from build123d import *

# Parameters (mm, degrees)
SKETCH_R   = 3
SKETCH_R_2 = 1.5
PAD_DEPTH  = 1.5


with BuildPart() as part:
    # Sketch → Pad (new body)
    with BuildSketch(Plane.XY):
        with BuildLine():
            Line((70, 0), (0, 0))
            Line((0, 0), (0, 50))
            Line((0, 50), (70, 50))
            Line((70, 50), (70, 40))
            ThreePointArc((70, 40), (55, 25), (70, 10))
            Line((70, 0), (70, 10))
        make_face()
        with Locations((28, 25)):
            Circle(SKETCH_R, mode=Mode.SUBTRACT)
        with Locations((49, 25)):
            Circle(SKETCH_R_2, mode=Mode.SUBTRACT)
        with Locations((59.5, 43.19)):
            Circle(SKETCH_R_2, mode=Mode.SUBTRACT)
        with Locations((59.5, 6.81)):
            Circle(SKETCH_R_2, mode=Mode.SUBTRACT)
    extrude(amount=PAD_DEPTH)


solid = part.part
CAD build for the part. Positions are in the model's coordinates, mm. Coordinates: 2 decimals unless noted, no trailing zeros. Write each loop counter-clockwise with the first axis right and the second up, starting at its lowest first coordinate (ties: lowest second). Pieces come first, ordered by that corner, then holes. Notation, with made-up numbers: M -18.5,83 L 19.5,83 A25 ccw 19.5,103 Z; hole C 11,28.5 d4. An arc over 180 degrees is marked long. Return JSON: item names as keys, results as strings.
Item 1: Slice it at B-B, the plane y = 6.81. Write the cut outline in (x, z), and give its area (4 significant figures).
Findings below:
{"outline": "M 0,0 L 58,0 L 58,1.5 L 0,1.5 Z; M 61,0 L 70,0 L 70,1.5 L 61,1.5 Z", "area": "100.5 mm2"}
Item 2: Probe line 1 (Y direction, x = 49, z = 0.65); line 2 (Y direction, x = 59.5, z = 0.85); line 3 (Y direction, x = 63.5, z = 0.55). List the from-to ranges inside material, lowest first. Write a range as from..to.
Findings below:
{"line 1": "y = 0..23.5, 26.5..50", "line 2": "y = 0..5.31, 8.31..14.29, 35.71..41.69, 44.69..50", "line 3": "y = 0..11.48, 38.52..50"}
Item 3: Two-plate mould, pull along Y, no slides. Class faces 1 (the flat face through (35, 50, 1)), 2 (the flat face through (35, 25, 0)), 3 (the cylindrical face through (60.93, 7.26, 0.74)), 4 (the cylindrical face through (60.886, 42.615, 0.74)): +Y half, -Y half, draft (parallel to the pull), parting line (faces both ways), or undercut.
Findings below:
{"face 1": "+Y half", "face 2": "draft", "face 3": "undercut", "face 4": "undercut"}
Item 4: Slice it at D-D, the plane x = 59.5. Write the cut outline in (y, z), and give its area (3 significant figures).
Findings below:
{"outline": "M 0,0 L 5.31,0 L 5.31,1.5 L 0,1.5 Z; M 8.31,0 L 14.29,0 L 14.29,1.5 L 8.31,1.5 Z; M 35.71,0 L 41.69,0 L 41.69,1.5 L 35.71,1.5 Z; M 44.69,0 L 50,0 L 50,1.5 L 44.69,1.5 Z", "area": "33.9 mm2"}
Item 5: Drop flat-ended pins along their axis: pin 1 Ø5 at (x, y) = (28, 25) entering from +Z; pin 2 Ø5 at (x, y) = (59.5, 43.19) entering from -Z. Give the stop position or say it passes through.
Findings below:
{"pin 1": "passes through", "pin 2": "stops at z = 0"}
Item 6: Slice it at A-A, the plane x = 49. Write the cut outline in (y, z), and give its area (3 significant figures).
Findings below:
{"outline": "M 0,0 L 23.5,0 L 23.5,1.5 L 0,1.5 Z; M 26.5,0 L 50,0 L 50,1.5 L 26.5,1.5 Z", "area": "70.5 mm2"}
Item 7: Slice it at C-C, the plane z = 0.5. Write the cut outline in (x, y).
Findings below:
{"outline": "M 0,0 L 70,0 L 70,10 A15 cw 70,40 L 70,50 L 0,50 Z; hole C 28,25 d6; hole C 49,25 d3; hole C 59.5,6.81 d3; hole C 59.5,43.19 d3"}
